```python
from build123d import *

# Parameters (mm, degrees)
SKETCH1_W           = 7
SKETCH1_H           = 20
BOSS_EXTRUDE2_DEPTH = 4
SKETCH1_4_R         = 0.925
SKETCH1_4_W         = 7
SKETCH1_4_H         = 20
BOSS_EXTRUDE3_DEPTH = 2
SKETCH1_5_R         = 0.925
BOSS_EXTRUDE4_DEPTH = 4
SKETCH1_6_R         = 3.155
BOSS_EXTRUDE5_DEPTH = 11.7
CUT_EXTRUDE1_DEPTH  = 4.85


with BuildPart() as part:
    # Sketch1 → Boss-Extrude2 (new body)
    with BuildSketch(Plane(origin=(0, 0, 0), x_dir=(1, 0, 0), z_dir=(0, 1, 0))):
        with Locations((-33.759922188, -0.124838084)):
            Rectangle(SKETCH1_W, SKETCH1_H)
    extrude(amount=BOSS_EXTRUDE2_DEPTH)

    # Sketch1<4> → Boss-Extrude3 (add)
    with BuildSketch(Plane(origin=(0, 0, 0), x_dir=(1, 0, 0), z_dir=(0, 1, 0))):
        with BuildLine():
            ThreePointArc((27.470986964, -10.749838084), (21.665077812, -0.124838084), (27.470986964, 10.500161916))
            Line((27.470986964, 10.500161916), (-48.259922188, 10.500161916))
            Line((-48.259922188, 10.500161916), (-48.259922188, -10.749838084))
            Line((-48.259922188, -10.749838084), (27.470986964, -10.749838084))
        make_face()
        with Locations((-16.839922188, -7.381359305)):
            Circle(SKETCH1_4_R, mode=Mode.SUBTRACT)
        with Locations((-33.759922188, -0.124838084)):
            Rectangle(SKETCH1_4_W, SKETCH1_4_H, mode=Mode.SUBTRACT)
        with Locations((-16.839922188, 5.570161916)):
            Circle(SKETCH1_4_R, mode=Mode.SUBTRACT)
        with BuildLine():
            Line((32.290077812, 10.500161916), (27.470986964, 10.500161916))
            ThreePointArc((27.470986964, 10.500161916), (21.665077812, -0.124838084), (27.470986964, -10.749838084))
            Line((27.470986964, -10.749838084), (32.290077812, -10.749838084))
            Line((32.290077812, -10.749838084), (32.290077812, 10.500161916))
        make_face()
        with Locations((30.160077812, -7.381359305)):
            Circle(SKETCH1_4_R, mode=Mode.SUBTRACT)
        with Locations((30.160077812, 5.570161916)):
            Circle(SKETCH1_4_R, mode=Mode.SUBTRACT)
    extrude(amount=BOSS_EXTRUDE3_DEPTH)

    # Sketch1<5> → Boss-Extrude4 (add)
    with BuildSketch(Plane(origin=(0, 0, 0), x_dir=(1, 0, 0), z_dir=(0, 1, 0))):
        with Locations((-16.839922188, 5.570161916)):
            Circle(SKETCH1_5_R)
        with Locations((-16.839922188, -7.381359305)):
            Circle(SKETCH1_5_R)
        with Locations((30.160077812, -7.381359305)):
            Circle(SKETCH1_5_R)
        with Locations((30.160077812, 5.570161916)):
            Circle(SKETCH1_5_R)
    extrude(amount=BOSS_EXTRUDE4_DEPTH)

    # Sketch1<6> → Boss-Extrude5 (add)
    with BuildSketch(Plane(origin=(0, 0, 0), x_dir=(1, 0, 0), z_dir=(0, 1, 0))):
        with BuildLine():
            Line((34.290077812, 12.500161916), (-50.259922188, 12.500161916))
            Line((-50.259922188, 12.500161916), (-50.259922188, -12.749838084))
            Line((-50.259922188, -12.749838084), (34.290077812, -12.749838084))
            ThreePointArc((34.290077812, -12.749838084), (30.736910211, -12.239524419), (27.470986964, -10.749838084))
            Line((27.470986964, -10.749838084), (-48.259922188, -10.749838084))
            Line((-48.259922188, -10.749838084), (-48.259922188, 10.500161916))
            Line((-48.259922188, 10.500161916), (27.470986964, 10.500161916))
            ThreePointArc((27.470986964, 10.500161916), (30.736910211, 11.989848251), (34.290077812, 12.500161916))
        make_face()
        with BuildLine():
            Line((34.290077812, -12.749838084), (34.290077812, 12.500161916))
            ThreePointArc((34.290077812, 12.500161916), (30.736910211, 11.989848251), (27.470986964, 10.500161916))
            Line((27.470986964, 10.500161916), (32.290077812, 10.500161916))
            Line((32.290077812, 10.500161916), (32.290077812, -10.749838084))
            Line((32.290077812, -10.749838084), (27.470986964, -10.749838084))
            ThreePointArc((27.470986964, -10.749838084), (30.736910211, -12.239524419), (34.290077812, -12.749838084))
        make_face()
        with BuildLine():
            ThreePointArc((46.915077812, -0.124838084), (43.217300925, 8.802385028), (34.290077812, 12.500161916))
            Line((34.290077812, 12.500161916), (34.290077812, -12.749838084))
            ThreePointArc((34.290077812, -12.749838084), (43.217300925, -9.052061197), (46.915077812, -0.124838084))
        make_face()
        with Locations((40.600077812, -0.124838084)):
            Circle(SKETCH1_6_R, mode=Mode.SUBTRACT)
    extrude(amount=BOSS_EXTRUDE5_DEPTH)

    # Sketch3 → Cut-Extrude1 (cut, symmetric)
    with BuildSketch(Plane.ZY.offset(50.259922188)):
        with BuildLine():
            Line((-2.800161916, 7.175), (3.049838084, 7.175))
            ThreePointArc((3.049838084, 7.175), (4.374838084, 5.85), (3.049838084, 4.525))
            Line((3.049838084, 4.525), (-2.800161916, 4.525))
            ThreePointArc((-2.800161916, 4.525), (-4.125161916, 5.85), (-2.800161916, 7.175))
        make_face()
    extrude(amount=CUT_EXTRUDE1_DEPTH, both=True, mode=Mode.SUBTRACT)


solid = part.part
```
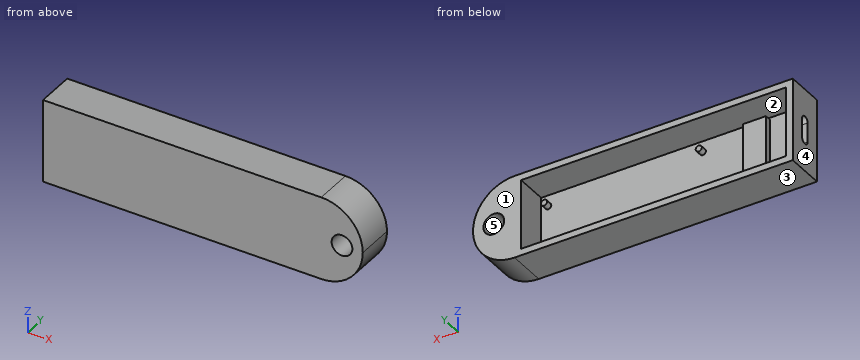
Could you check a few things on this model? Use its own coordinates, in mm. Face numbers are marked on the shaded views. A direction names the side the tool comes from. Round coordinates to 2 decimals unless told otherwise and drop trailing zeros. Loops run counter-clockwise (first coordinate to the right, second up) from the corner with the lowest first, then second, coordinate; pieces in that order, holes last.
Q1. On a 3-axis mill with a long thin cutter (end or side, diameter ignored), from which of +Z, -Z, +X, -X, +Y, -Y can I reach the whole of each face in a straight line? I mean the marked faces 1 and 2. Say none if no direction works.
Q2. Thinking about a two-plate mould opening in Z: for the marked faces 3, 4 and 5, which applies, pulls with the +Z half, pulls with the -Z half, needs draft (parallel to the pull), parting line crosses it, or undercut?
Q3. For P1, Ø8, axis at x = -29, z = 4.5, coming from the +Y side; P2, Ø2, axis at y = 2.5, z = -1.5, coming from the +X side; P3, Ø4, axis at x = 40.6, z = 0.12, coming from the -Y side (3 decimals); P4, Ø5, axis at y = 8.5, z = 8, coming from the +X side, each with a flat end and sliding along its axis, tell me the tip position at first contact or that it passes through.
Q4. I want a section at B-B (y = 5.85). Write out the boundary of the cut face in (x, z) (3 decimals).
Q5. I want a section at A-A (x = -29). Write out the boundary of the cut face in (y, z), and give its area (3 significant figures).
Q6. I want a section at C-C (z = 1.5). Write out the boundary of the cut face in (x, y) (3 decimals), and give its area (3 significant figures).
Q7. Please list where these lines run through material, in increasing order: L1, parallel to X at y = 3, z = 7.5; L2, parallel to Z at x = 4, y = 4; L3, parallel to X at y = 11, z = 0.5.
Answer below:
1. face 1: +Z, -Z, +X, -X, +Y
1. face 2: +Y
2. face 3: pulls with the -Z half
2. face 4: needs draft
2. face 5: undercut
3. P1: stops at y = 4
3. P2: stops at x = 46.9
3. P3: passes through
3. P4: stops at x = 45.71
4. outline: (-50.26, -12.5) - (34.29, -12.5) arc R12.625 ccw to (34.29, 12.75) - (-50.26, 12.75) - (-50.26, 4.375) - (-48.26, 4.375) - (-48.26, 10.75) - (32.29, 10.75) - (32.29, -10.5) - (-48.26, -10.5) - (-48.26, -4.125) - (-50.26, -4.125) - close; hole circle Ø6.31 at (40.6, 0.125)
5. outline: (0, -12.5) - (11.7, -12.5) - (11.7, -10.5) - (2, -10.5) - (2, 10.75) - (11.7, 10.75) - (11.7, 12.75) - (0, 12.75) - close
5. area: 89.3 mm2
6. outline: (-50.26, 0) - (37.761, 0) - (37.761, 11.7) - (32.29, 11.7) - (32.29, 2) - (-30.26, 2) - (-30.26, 4) - (-37.26, 4) - (-37.26, 2) - (-48.26, 2) - (-48.26, 4.525) - (-50.26, 4.525) - close; (-50.26, 7.175) - (-48.26, 7.175) - (-48.26, 11.7) - (-50.26, 11.7) - close; (43.44, 0) - (46.84, 0) - (46.84, 11.7) - (43.44, 11.7) - close
6. area: 297 mm2
7. L1: x = -50.26 to -48.26, -37.26 to -30.26, -17.76 to -15.92, 29.24 to 31.08, 32.29 to 44.54
7. L2: z = -12.5 to -10.5, 10.75 to 12.75
7. L3: x = -50.26 to -48.26, 32.29 to 37.47, 43.73 to 46.91
